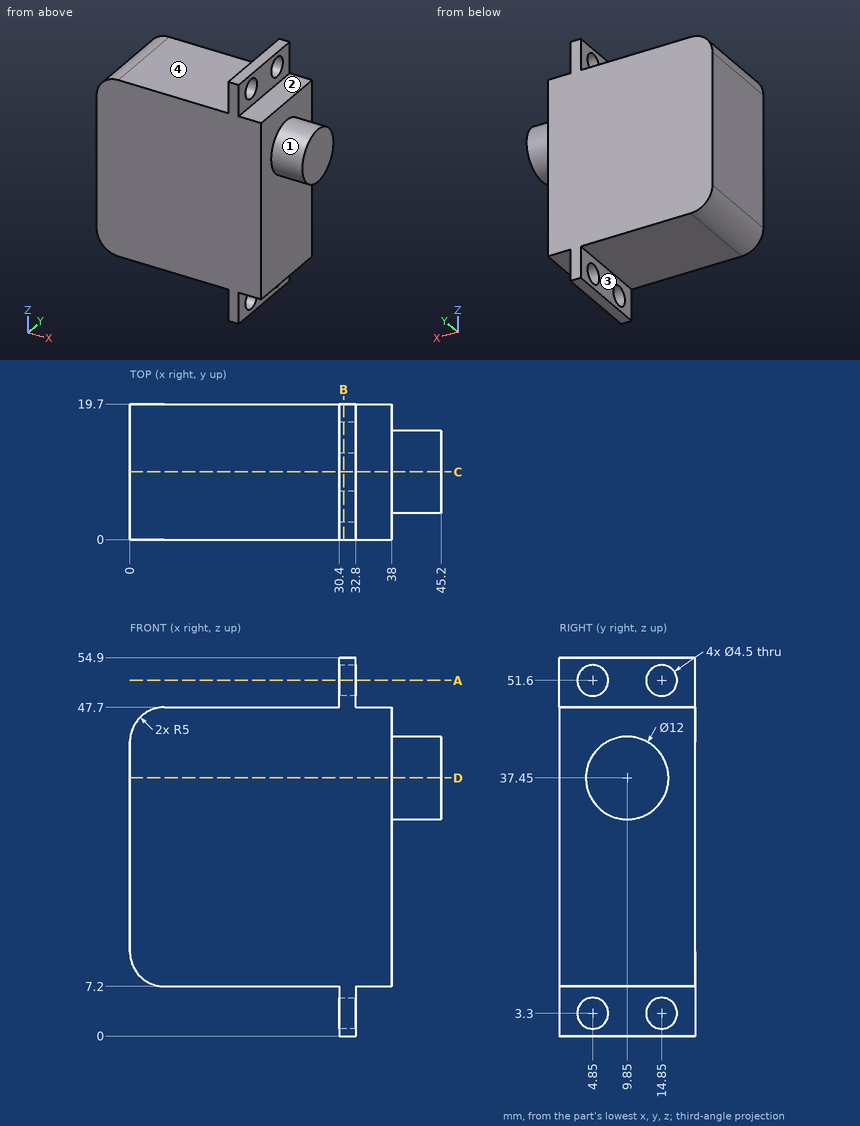
Study the drawing (mm; zero at the part's minimum x, y, z) and answer. A direction names the side the tool comes from. Coordinates: 2 decimals unless noted, no trailing zeros. Write each loop counter-clockwise with the first axis right and the second up, starting at its lowest first coordinate (ties: lowest second). Pieces come first, ordered by that corner, then holes. Notation, with made-up numbers: M 10.5,59 L 62.5,59 A27 ccw 62.5,76 Z; hole C -33.75,67.25 d10. An arc over 180 degrees is marked long. Use a Markdown table: item, result. Add a question column.
1. Section A-A (z = 51.6) is taken. Give the vertices of the cut face in (x, y), plus the area to 3 significant figures.
2. Section D-D (z = 37.45) is taken. Give the vertices of the cut face in (x, y), plus the area to 3 significant figures.
3. Given P1, Ø4, axis at x = 35, y = 5.5, coming from the -Z side; P2, Ø7, axis at y = 4.85, z = 3.3, coming from the -X side; P3, Ø5, axis at y = 4.85, z = 51.6, coming from the +X side; P4, Ø1, axis at x = 36, z = 17.5, coming from the -Y side, each flat-ended and moving along its own axis, determine where each tip first touches the part or whether it passes through.
4. Section B-B (x = 31) is taken. Give the vertices of the cut face in (y, z).
5. Straight lines are drawn through the part: line 1 along Y through (x, z) = (31.2, 51.6); line 2 along X through (y, z) = (6.75, 21); line 3 along Z through (x, y) = (27.5, 10.25). For each, find the intervals that lie inside material, in ascending order. Write a range as [from, to].
6. Which of the six approach directions +Z, -Z, +X, -X, +Y, -Y give full straight-line access (tool end or side, diameter ignored) to the marked faces 1, 2, 3 and 4?
7. Section C-C (y = 9.85) is taken. Give the vertices of the cut face in (x, z).
Data:
| question | item | result |
|---|---|---|
| 1 | outline | M 30.4,0 L 32.8,0 L 32.8,2.6 L 30.4,2.6 Z; M 30.4,7.1 L 32.8,7.1 L 32.8,12.6 L 30.4,12.6 Z; M 30.4,17.1 L 32.8,17.1 L 32.8,19.7 L 30.4,19.7 Z |
| 1 | area | 25.7 mm2 |
| 2 | outline | M 0,0 L 38,0 L 38,3.85 L 45.2,3.85 L 45.2,15.85 L 38,15.85 L 38,19.7 L 0,19.7 Z |
| 2 | area | 835 mm2 |
| 3 | P1 | stops at z = 7.2 |
| 3 | P2 | stops at x = 30.4 |
| 3 | P3 | stops at x = 32.8 |
| 3 | P4 | stops at y = 0 |
| 4 | outline | M 0,0 L 19.7,0 L 19.7,54.9 L 0,54.9 Z; hole C 4.85,3.3 d4.5; hole C 4.85,51.6 d4.5; hole C 14.85,3.3 d4.5; hole C 14.85,51.6 d4.5 |
| 5 | line 1 | y = [0, 2.6], [7.1, 12.6], [17.1, 19.7] |
| 5 | line 2 | x = [0, 38] |
| 5 | line 3 | z = [7.2, 47.7] |
| 6 | face 1 | +X |
| 6 | face 2 | +Z, +X, +Y, -Y |
| 6 | face 3 | -Z, -X, +Y, -Y |
| 6 | face 4 | +Z, -X, +Y, -Y |
| 7 | outline | M 0,12.2 A5 ccw 5,7.2 L 30.4,7.2 L 30.4,0 L 32.8,0 L 32.8,7.2 L 38,7.2 L 38,31.45 L 45.2,31.45 L 45.2,43.45 L 38,43.45 L 38,47.7 L 32.8,47.7 L 32.8,54.9 L 30.4,54.9 L 30.4,47.7 L 5,47.7 A5 ccw 0,42.7 Z |
